For this review, take the finished solid that the model builds, in its own axes (mm). Give positions to 0.01 mm unless a question says otherwise; leave off trailing zeros. Loops run counter-clockwise (first coordinate to the right, second up) from the corner with the lowest first, then second, coordinate; pieces in that order, holes last.
```python
from build123d import *

# Parameters (mm, degrees)
SKETCH1_W            = 28
SKETCH1_H            = 22
BOSS_EXTRUDE1_DEPTH  = 1.27
SKETCH2_R            = 1.2999974
CUT_EXTRUDE2_DEPTH   = 2.27
LPATTERN1_COUNT      = 2
LPATTERN1_PITCH      = 11
LPATTERN1_COUNT_DIR2 = 2
LPATTERN1_PITCH_DIR2 = 16


with BuildPart() as part:
    # Sketch1 → Boss-Extrude1 (new body)
    with BuildSketch(Plane(origin=(0, 0, 0), x_dir=(1, 0, 0), z_dir=(0, 1, 0))):
        Rectangle(SKETCH1_W, SKETCH1_H)
    extrude(amount=BOSS_EXTRUDE1_DEPTH)

    # Sketch2 → Cut-Extrude2 (cut, through all)
    with BuildSketch(Plane(origin=(0, 0, 0), x_dir=(1, 0, 0), z_dir=(0, 1, 0))):
        with Locations((-11, 8)):
            Circle(SKETCH2_R)
    cut_extrude2 = extrude(amount=CUT_EXTRUDE2_DEPTH, mode=Mode.SUBTRACT)

    # LPattern1: Cut-Extrude2 2 × 2
    with Locations(*[(i * LPATTERN1_PITCH, 0, j * LPATTERN1_PITCH_DIR2) for i in range(LPATTERN1_COUNT) for j in range(LPATTERN1_COUNT_DIR2) if (i, j) != (0, 0)]):
        add(cut_extrude2, mode=Mode.SUBTRACT)


solid = part.part
```
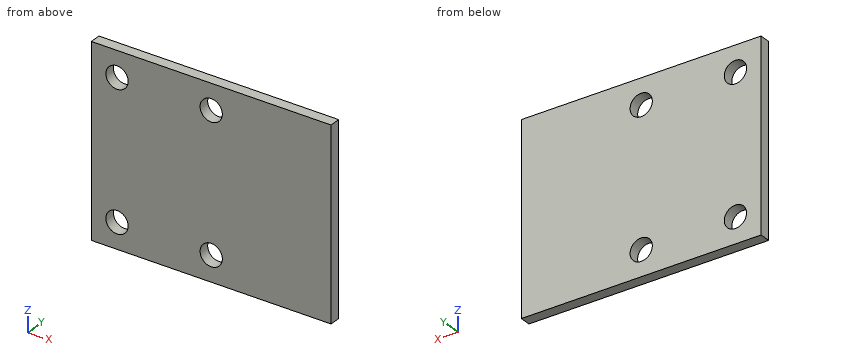
Q1. For pin 1 Ø10 at (x, z) = (2.5, -8) entering from -Y, flat-tipped, find the tip position at first contact; note if it passes through.
Answers:
pin 1: stops at y = 0
Q2. For probe 1 along Z at (x, y) = (-11, 0.5); probe 2 along X at (y, z) = (0.35, -8); probe 3 along Z at (x, y) = (-0.5, 0.4), list the stretches that pass through material, from the lowest coordinate up.
Answers:
probe 1: z = -11 to -9.3, -6.7 to 6.7, 9.3 to 11
probe 2: x = -14 to -12.3, -9.7 to -1.3, 1.3 to 14
probe 3: z = -11 to -9.2, -6.8 to 6.8, 9.2 to 11
Q3. Consider section A-A on x = 0. Give the boundary of the cut face in (y, z).
Answers:
outline: (0, -11) - (1.27, -11) - (1.27, -9.3) - (0, -9.3) - close; (0, -6.7) - (1.27, -6.7) - (1.27, 6.7) - (0, 6.7) - close; (0, 9.3) - (1.27, 9.3) - (1.27, 11) - (0, 11) - close
Q4. Consider section B-B on y = 0.2. Give the boundary of the cut face in (x, z), plus the area to 3 significant figures.
Answers:
outline: (-14, -11) - (14, -11) - (14, 11) - (-14, 11) - close; hole circle Ø2.6 at (-11, -8); hole circle Ø2.6 at (-11, 8); hole circle Ø2.6 at (0, -8); hole circle Ø2.6 at (0, 8)
area: 595 mm2
Q5. Consider section C-C on z = -8. Give the boundary of the cut face in (x, y), plus the area to 3 significant figures.
Answers:
outline: (-14, 0) - (-12.3, 0) - (-12.3, 1.27) - (-14, 1.27) - close; (-9.7, 0) - (-1.3, 0) - (-1.3, 1.27) - (-9.7, 1.27) - close; (1.3, 0) - (14, 0) - (14, 1.27) - (1.3, 1.27) - close
area: 29.0 mm2
